Could you check a few things on this model? Use its own coordinates, in mm. A direction names the side the tool comes from. Round coordinates to 2 decimals unless told otherwise and drop trailing zeros. Write each loop counter-clockwise with the first axis right and the second up, starting at its lowest first coordinate (ties: lowest second). Pieces come first, ordered by that corner, then holes. Notation, with made-up numbers: (9.5, 40) -> (66.5, 40) arc R28 ccw to (66.5, 62) -> close; hole circle Ø1 at (66.25, 66.25). An arc over 180 degrees is marked (long way). Answer as CSV lines item,"result". Start each with the question number.
Q1. Imagine slicing it at A-A on z = -23.5. Give the number of separate pieces and of enclosed holes in the cut face, and give its area (3 significant figures).
Q2. If I drill on line 1 (X direction, y = 7.25, z = -68.75); line 2 (Z direction, x = -30, y = 6.25); line 3 (X direction, y = 28.5, z = -77), over which ranges is the centre line in solid material (lowest first)? Write a range as [from, to].
Q3. Imagine slicing it at B-B on x = 22. Please give me the cut outline in (y, z), and give its area (3 significant figures).
Q4. Imagine slicing it at D-D on y = 31.5. Please give me the cut outline in (x, z).
Q5. For faces 4 (the cylindrical face through (0, 6, -5)), 5 (the flat face through (36.512, 17, -41)), 6 (the flat face through (32, 14, -14)), 7 (the flat face through (-39, 17, -24)), which set-ups out of +Z, -Z, +X, -X, +Y, -Y let a thin tool reach every point of the face, with its end or its side?
Q6. Will these pins go through, and if not, where does the flat tip stop? pin 1 Ø12.5 at (y, z) = (21, -22.5) entering from -X; pin 2 Ø2.5 at (x, z) = (31, -13) entering from +Y.
Q7. If we mould it in two halves opening along Z, with no side actions, what happens to faces 1 (the flat face through (-1, 9, 0)), 2 (the flat face through (38.86, 25.67, -54.54)), 3 (the flat face through (40, 34, -42))? For each: pulls with the +Z half, pulls with the -Z half, needs draft (parallel to the pull), parting line crosses it, or undercut.
Q8. Imagine slicing it at C-C on z = -68.75. Please give me the cut outline in (x, y).
from build123d import *

# Parameters (mm, degrees)
SKETCH1_W                   = 89
SKETCH1_H                   = 83
SKETCH1_R                   = 1.3
MAIN_BODY_DEPTH             = 14
SKETCH2_W                   = 73.025
SKETCH2_H                   = 83
SKETCH2_R                   = 4
SCREW_RISER_DEPTH           = 2
SKETCH4_W                   = 7.9875
SKETCH4_H                   = 83
TOPPER_SUPPORT_DEPTH        = 20
MOUNT_START                 = -44.5
MOUNT_NUTS_DEPTH            = 41.275
F_9_32_MOUNT_HOLES_REACH    = 9.988
SKETCH5_R                   = 3.3734375
SKETCH8_W                   = 19.0125
SKETCH8_H                   = 43
MIDDLE_CUT_DEPTH            = 14
SKETCH9_R                   = 3.3734375
MOUNT_NUTS_P2_DEPTH         = 4.7625
SKETCH9_3_R                 = 3.3734375
F_9_32_MOUNT_HOLES_P2_DEPTH = 7.9875


with BuildPart() as part:
    # Sketch1 → Main Body (new body)
    with BuildSketch(Plane(origin=(0, 0, 0), x_dir=(1, 0, 0), z_dir=(0, 1, 0))):
        with Locations((0, 41.5)):
            Rectangle(SKETCH1_W, SKETCH1_H)
        with Locations((-30, 14.25)):
            Circle(SKETCH1_R, mode=Mode.SUBTRACT)
        with Locations((30, 14.25)):
            Circle(SKETCH1_R, mode=Mode.SUBTRACT)
        with BuildLine():
            Line((-7.5, 12.5), (-7.5, 70.5))
            ThreePointArc((-7.5, 70.5), (0, 78), (7.5, 70.5))
            Line((7.5, 70.5), (7.5, 12.5))
            ThreePointArc((7.5, 12.5), (0, 5), (-7.5, 12.5))
        make_face(mode=Mode.SUBTRACT)
        with Locations((-30, 68.75)):
            Circle(SKETCH1_R, mode=Mode.SUBTRACT)
        with Locations((30, 68.75)):
            Circle(SKETCH1_R, mode=Mode.SUBTRACT)
    extrude(amount=MAIN_BODY_DEPTH)

    # Sketch2 → Screw Riser (cut)
    with BuildSketch(Plane(origin=(0, 14, 0), x_dir=(1, 0, 0), z_dir=(0, 1, 0))):
        with Locations((0, 41.5)):
            Rectangle(SKETCH2_W, SKETCH2_H)
        with Locations((-30, 14.25)):
            Circle(SKETCH2_R, mode=Mode.SUBTRACT)
        with Locations((30, 14.25)):
            Circle(SKETCH2_R, mode=Mode.SUBTRACT)
        with Locations((-30, 68.75)):
            Circle(SKETCH2_R, mode=Mode.SUBTRACT)
        with Locations((30, 68.75)):
            Circle(SKETCH2_R, mode=Mode.SUBTRACT)
    extrude(amount=-SCREW_RISER_DEPTH, mode=Mode.SUBTRACT)

    # Sketch4 → Topper Support (add)
    with BuildSketch(Plane(origin=(0, 14, 0), x_dir=(1, 0, 0), z_dir=(0, 1, 0))):
        with Locations((-40.50625, 41.5)):
            Rectangle(SKETCH4_W, SKETCH4_H)
        with Locations((40.50625, 41.5)):
            Rectangle(SKETCH4_W, SKETCH4_H)
    extrude(amount=TOPPER_SUPPORT_DEPTH)

    # Sketch6 → Mount Nuts (cut)
    with BuildSketch(Plane.ZY.offset(44.5).offset(MOUNT_START)):
        Polygon((-52.855059246, 22.7546875), (-56.177529623, 28.509375), (-62.822470377, 28.509375), (-66.144940754, 22.7546875), (-62.822470377, 17), (-56.177529623, 17), align=None)
        Polygon((-16.855059246, 22.7546875), (-20.177529623, 28.509375), (-26.822470377, 28.509375), (-30.144940754, 22.7546875), (-26.822470377, 17), (-20.177529623, 17), align=None)
    extrude(amount=MOUNT_NUTS_DEPTH, mode=Mode.SUBTRACT)

    # Sketch5 → 9/32 Mount Holes (cut, up to next)
    with BuildSketch(Plane.ZY.offset(36.5125), mode=Mode.PRIVATE) as f_9_32_mount_holes_sk1:
        with Locations((-59.5, 22.7546875)):
            Circle(SKETCH5_R)
    f_9_32_mount_holes_tool1 = extrude(f_9_32_mount_holes_sk1.sketch, amount=F_9_32_MOUNT_HOLES_REACH, mode=Mode.PRIVATE) & part.part
    add(f_9_32_mount_holes_tool1.solids().sort_by_distance((-36.5125, 22.754688, -59.5))[0], mode=Mode.SUBTRACT)
    # Sketch5 → 9/32 Mount Holes (cut, up to next)
    with BuildSketch(Plane.ZY.offset(36.5125), mode=Mode.PRIVATE) as f_9_32_mount_holes_sk2:
        with Locations((-23.5, 22.7546875)):
            Circle(SKETCH5_R)
    f_9_32_mount_holes_tool2 = extrude(f_9_32_mount_holes_sk2.sketch, amount=F_9_32_MOUNT_HOLES_REACH, mode=Mode.PRIVATE) & part.part
    add(f_9_32_mount_holes_tool2.solids().sort_by_distance((-36.5125, 22.754688, -23.5))[0], mode=Mode.SUBTRACT)

    # Sketch8 → Middle Cut (cut)
    with BuildSketch(Plane(origin=(0, 14, 0), x_dir=(1, 0, 0), z_dir=(0, 1, 0))):
        with Locations((-27.00625, 41.5)):
            Rectangle(SKETCH8_W, SKETCH8_H)
        with Locations((27.00625, 41.5)):
            Rectangle(SKETCH8_W, SKETCH8_H)
    extrude(amount=-MIDDLE_CUT_DEPTH, mode=Mode.SUBTRACT)

    # Sketch9 → Mount Nuts p2 (cut)
    with BuildSketch(Plane.ZY.offset(-36.5125)):
        Polygon((-56.177529623, 17), (-62.822470377, 17), (-66.144940754, 22.7546875), (-62.822470377, 28.509375), (-56.177529623, 28.509375), (-52.855059246, 22.7546875), align=None)
        with Locations((-59.5, 22.7546875)):
            Circle(SKETCH9_R, mode=Mode.SUBTRACT)
        with Locations((-59.5, 22.7546875)):
            Circle(SKETCH9_R)
        Polygon((-20.177529623, 17), (-26.822470377, 17), (-30.144940754, 22.7546875), (-26.822470377, 28.509375), (-20.177529623, 28.509375), (-16.855059246, 22.7546875), align=None)
        with Locations((-23.5, 22.7546875)):
            Circle(SKETCH9_R, mode=Mode.SUBTRACT)
        with Locations((-23.5, 22.7546875)):
            Circle(SKETCH9_R)
    extrude(amount=-MOUNT_NUTS_P2_DEPTH, mode=Mode.SUBTRACT)

    # Sketch9<3> → 9/32 Mount Holes p2 (cut)
    with BuildSketch(Plane.ZY.offset(-36.5125)):
        with Locations((-59.5, 22.7546875)):
            Circle(SKETCH9_3_R)
        with Locations((-23.5, 22.7546875)):
            Circle(SKETCH9_3_R)
    extrude(amount=-F_9_32_MOUNT_HOLES_P2_DEPTH, mode=Mode.SUBTRACT)


solid = part.part
Checks:
1,separate pieces,"6"
1,enclosed holes,"0"
1,area,"630 mm^2"
2,line 1,"[-44.5, -31.3], [-28.7, -7.5], [7.5, 28.7], [31.3, 44.5]"
2,line 2,"[-83, -70.05], [-67.45, -63], [-20, -15.55], [-12.95, 0]"
2,line 3,"[-44.5, -36.51], [36.51, 44.5]"
3,outline,"(0, -83) -> (12, -83) -> (12, -63) -> (0, -63) -> close; (0, -20) -> (12, -20) -> (12, 0) -> (0, 0) -> close"
3,area,"480 mm^2"
4,outline,"(-44.5, -83) -> (-36.51, -83) -> (-36.51, 0) -> (-44.5, 0) -> close; (36.51, -83) -> (44.5, -83) -> (44.5, 0) -> (36.51, 0) -> close"
5,face 4,"+Y, -Y"
5,face 5,"+Y"
5,face 6,"+Z, -Z, +Y"
5,face 7,"none"
6,pin 1,"x = -44.5"
6,pin 2,"y = 14"
7,face 1,"pulls with the +Z half"
7,face 2,"undercut"
7,face 3,"needs draft"
8,outline,"(-44.5, 0) -> (-31.3, 0) -> (-31.3, 14) -> (-34, 14) -> (-34, 12) -> (-36.51, 12) -> (-36.51, 34) -> (-44.5, 34) -> close; (-28.7, 0) -> (-7.5, 0) -> (-7.5, 12) -> (-26, 12) -> (-26, 14) -> (-28.7, 14) -> close; (7.5, 0) -> (28.7, 0) -> (28.7, 14) -> (26, 14) -> (26, 12) -> (7.5, 12) -> close; (31.3, 0) -> (44.5, 0) -> (44.5, 34) -> (36.51, 34) -> (36.51, 12) -> (34, 12) -> (34, 14) -> (31.3, 14) -> close"
